from build123d import *

# Parameters (mm, degrees)
SKETCH1_R           = 1
SKETCH1_R_2         = 1.45
BOSS_EXTRUDE1_DEPTH = 1.5


with BuildPart() as part:
    # Sketch1 → Boss-Extrude1 (new body)
    with BuildSketch(Plane.XY):
        with BuildLine():
            Line((1, 0), (29, 0))
            ThreePointArc((29, 0), (29.707106781, 0.292893219), (30, 1))
            Line((30, 1), (30, 10.010805278))
            add(Edge.make_bspline(
                [(30, 10.010805278), (30, 10.331309343), (29.969485344, 10.646616833), (29.849948512, 11.267268119), (29.75966755, 11.575507617), (29.52283644, 12.166717494), (29.377858407, 12.44760172), (29.03567781, 12.980427757), (28.836063124, 13.234342382), (28.398424751, 13.693093363), (28.159679219, 13.900081722), (27.642024265, 14.268934545), (27.362921955, 14.429904426), (26.787626221, 14.692448411), (26.488674786, 14.796208342), (25.867413661, 14.94687591), (25.550156827, 14.992309833), (25.229989605, 15.007057677)],
                knots=[0, 0, 0, 0, 0.125, 0.125, 0.25, 0.25, 0.375, 0.375, 0.5, 0.5, 0.625, 0.625, 0.75, 0.75, 0.875, 0.875, 1, 1, 1, 1], degree=3))
            add(Edge.make_bspline(
                [(19.763139721, 20), (19.763139721, 15.258876858), (25.229989605, 15.007057677)],
                knots=[0, 0, 0, 1.517657498, 1.517657498, 1.517657498], degree=2, weights=[1, 0.725642413, 1]))
            Line((19.763139721, 20), (19.763139721, 65))
            Line((19.763139721, 65), (10.236860279, 65))
            Line((10.236860279, 65), (10.236860279, 20))
            add(Edge.make_bspline(
                [(4.770010395, 15.007057677), (10.236860279, 15.258876858), (10.236860279, 20)],
                knots=[4.765527809, 4.765527809, 4.765527809, 6.283185307, 6.283185307, 6.283185307], degree=2, weights=[1, 0.725642413, 1]))
            add(Edge.make_bspline(
                [(4.770010395, 15.007057677), (4.449845357, 14.992309934), (4.136282013, 14.947292066), (3.521812442, 14.799220851), (3.218062701, 14.694770205), (2.638478447, 14.430814604), (2.364622125, 14.272965812), (1.848237929, 13.906408033), (1.60386949, 13.695209671), (1.16596165, 13.236750613), (0.970282062, 12.988644641), (0.625834171, 12.454385704), (0.478004619, 12.168149386), (0.242397802, 11.581322908), (0.15257366, 11.277880984), (0.03075096, 10.650270556), (0, 10.331307007), (0, 10.010805278)],
                knots=[0, 0, 0, 0, 0.125, 0.125, 0.25, 0.25, 0.375, 0.375, 0.5, 0.5, 0.625, 0.625, 0.75, 0.75, 0.875, 0.875, 1, 1, 1, 1], degree=3))
            Line((0, 10.010805278), (0, 1))
            ThreePointArc((0, 1), (0.292893219, 0.292893219), (1, 0))
        make_face()
        with Locations((15, 4)):
            Circle(SKETCH1_R, mode=Mode.SUBTRACT)
        with Locations((15, 20)):
            Circle(SKETCH1_R_2, mode=Mode.SUBTRACT)
        with Locations((15, 35)):
            Circle(SKETCH1_R_2, mode=Mode.SUBTRACT)
    extrude(amount=BOSS_EXTRUDE1_DEPTH)


solid = part.part
Read the model definition and answer for the solid it produces. Units are mm, in the model's axes. A direction names the side the tool comes from. Coordinates: 2 decimals unless noted, no trailing zeros. Loops run counter-clockwise (first coordinate to the right, second up) from the corner with the lowest first, then second, coordinate; pieces in that order, holes last.
Q1. Each of these flat-tipped pins is pushed along its axis until it touches: pin 1 Ø0.8 at (y, z) = (33, 1) entering from -X; pin 2 Ø0.8 at (y, z) = (53, 0.5) entering from +X. Where does it stop, or does it pass through?
Q2. The part is cut by section C-C on y = 35. Write down the section's boundary in (x, z), and give its area (3 significant figures).
Q3. Which of the six approach directions +Z, -Z, +X, -X, +Y, -Y give full straight-line access (tool end or side, diameter ignored) to faces 4 (the face through (19.763, 42, 1)), 5 (the face through (10.237, 43, 1)), 6 (the face through (30, 5, 1))?
Q4. The part is cut by section B-B on z = 1. Give the number of separate pieces and of enclosed holes in the cut face, and give its area (3 significant figures).
Q5. Consider probe 1 along Y at (x, z) = (15, 0.9); probe 2 along X at (y, z) = (30.5, 0.7); probe 3 along X at (y, z) = (19, 0.95). Determine where each line is inside the solid, lowest interval first.
Q6. The mould has two halves that part along Y. Classify faces 1 (the face through (15, 0, 1)), 2 (the face through (0, 6, 1)), 3 (the face through (16, 4, 1)): +Y half, -Y half, draft (parallel to the pull), parting line (faces both ways), or undercut.
Q7. The part is cut by section A-A on y = 4. Write down the section's boundary in (x, z).
Q8. The part is cut by section D-D on y = 43. Write down the section's boundary in (x, z).
Results below:
1. pin 1: stops at x = 10.24
1. pin 2: stops at x = 19.76
2. outline: (10.24, 0) - (13.55, 0) - (13.55, 1.5) - (10.24, 1.5) - close; (16.45, 0) - (19.76, 0) - (19.76, 1.5) - (16.45, 1.5) - close
2. area: 9.94 mm2
3. face 4: +Z, -Z, +X, +Y
3. face 5: +Z, -Z, -X, +Y
3. face 6: +Z, -Z, +X, +Y, -Y
4. separate pieces: 1
4. enclosed holes: 3
4. area: 911 mm2
5. probe 1: y = 0 to 3, 5 to 18.55, 21.45 to 33.55, 36.45 to 65
5. probe 2: x = 10.24 to 19.76
5. probe 3: x = 10.12 to 13.95, 16.05 to 19.88
6. face 1: -Y half
6. face 2: draft
6. face 3: undercut
7. outline: (0, 0) - (14, 0) - (14, 1.5) - (0, 1.5) - close; (16, 0) - (30, 0) - (30, 1.5) - (16, 1.5) - close
8. outline: (10.24, 0) - (19.76, 0) - (19.76, 1.5) - (10.24, 1.5) - close
